from build123d import *

# Parameters (mm, degrees)
SKIZZE1_R                                            = 8
AUFSATZ_LINEAR_AUSTRAGEN1_DEPTH                      = 5
AUFSATZ_LINEAR_AUSTRAGEN2_DEPTH                      = 7.5
FORMSENKUNG_F_R_M3_SENKSCHRAUBE_MIT_SCHL_D           = 3.2
FORMSENKUNG_F_R_M3_SENKSCHRAUBE_MIT_SCHL_CSINK_D     = 6.3
FORMSENKUNG_F_R_M3_SENKSCHRAUBE_MIT_SCHL_CSINK_ANGLE = 90
M4_GEWINDEBOHRUNG2_D                                 = 3.3
M4_GEWINDEBOHRUNG2_DEPTH                             = 13
M4_GEWINDEBOHRUNG2_TIP                               = 0.991420021
SKIZZE15_R                                           = 18.25
SCHNITT_LINEAR_AUSTRAGEN1_DEPTH                      = 1
SKIZZE16_R                                           = 11.0125
SCHNITT_LINEAR_AUSTRAGEN2_DEPTH                      = 2.5


with BuildPart() as part:
    # Skizze1 → Aufsatz-Linear austragen1 (new body)
    with BuildSketch(Plane.XY):
        with BuildLine():
            Line((0, 0), (52.5, 0))
            Line((52.5, 0), (52.5, 7.5))
            Line((52.5, 7.5), (48.11327046, 38.207106781))
            ThreePointArc((48.11327046, 38.207106781), (46.439531698, 41.277269775), (43.163522992, 42.5))
            Line((43.163522992, 42.5), (9.336477008, 42.5))
            ThreePointArc((9.336477008, 42.5), (6.060468302, 41.277269775), (4.38672954, 38.207106781))
            Line((4.38672954, 38.207106781), (0, 7.5))
            Line((0, 7.5), (0, 0))
        make_face()
        with Locations((26.25, 21.25)):
            Circle(SKIZZE1_R, mode=Mode.SUBTRACT)
    extrude(amount=AUFSATZ_LINEAR_AUSTRAGEN1_DEPTH)

    # Skizze4 → Aufsatz-Linear austragen2 (add)
    with BuildSketch(Plane.XZ):
        with BuildLine():
            Line((52.5, 0), (47.5, 0))
            Line((47.5, 0), (47.5, -7.5))
            ThreePointArc((47.5, -7.5), (50, -10), (52.5, -7.5))
            Line((52.5, -7.5), (52.5, 0))
        make_face()
        with BuildLine():
            Line((0, 0), (5, 0))
            Line((5, 0), (5, -7.5))
            ThreePointArc((5, -7.5), (2.5, -10), (0, -7.5))
            Line((0, -7.5), (0, 0))
        make_face()
    extrude(amount=-AUFSATZ_LINEAR_AUSTRAGEN2_DEPTH)

    # Formsenkung für M3 Senkschraube mit Schlitz/Kreuzschlitz1 (through all)
    with Locations(Plane.XY.offset(5)):
        with Locations((16.350505063, 31.149494937), (36.149494937, 11.350505063), (16.350505063, 11.350505063), (36.149494937, 31.149494937)):
            CounterSinkHole(FORMSENKUNG_F_R_M3_SENKSCHRAUBE_MIT_SCHL_D / 2, FORMSENKUNG_F_R_M3_SENKSCHRAUBE_MIT_SCHL_CSINK_D / 2, counter_sink_angle=FORMSENKUNG_F_R_M3_SENKSCHRAUBE_MIT_SCHL_CSINK_ANGLE)

    # M4 Gewindebohrung2
    with Locations(Plane(origin=(0, 0, 0), x_dir=(-1, 0, 0), z_dir=(0, -1, 0))):
        with Locations((-2.5, 7.5), (-50, 7.5), (-50, -2.5), (-2.5, -2.5)):
            Hole(M4_GEWINDEBOHRUNG2_D / 2, depth=M4_GEWINDEBOHRUNG2_DEPTH)
            with Locations((0, 0, -(M4_GEWINDEBOHRUNG2_DEPTH + M4_GEWINDEBOHRUNG2_TIP / 2))):  # 118° drill point
                Cone(0, M4_GEWINDEBOHRUNG2_D / 2, M4_GEWINDEBOHRUNG2_TIP, mode=Mode.SUBTRACT)

    # Skizze15 → Schnitt-Linear austragen1 (cut)
    with BuildSketch(Plane(origin=(0, 0, 0), x_dir=(-1, 0, 0), z_dir=(0, 0, -1))):
        with Locations((-26.25, 21.25)):
            Circle(SKIZZE15_R)
    extrude(amount=-SCHNITT_LINEAR_AUSTRAGEN1_DEPTH, mode=Mode.SUBTRACT)

    # Skizze16 → Schnitt-Linear austragen2 (cut)
    with BuildSketch(Plane(origin=(0, 0, 1), x_dir=(-1, 0, 0), z_dir=(0, 0, -1))):
        with Locations((-26.25, 21.25)):
            Circle(SKIZZE16_R)
    extrude(amount=-SCHNITT_LINEAR_AUSTRAGEN2_DEPTH, mode=Mode.SUBTRACT)


solid = part.part
Source: CAD feature listing. Evaluate the final solid. Frame: model axes, mm. A direction names the side the tool comes from. Give positions to 0.01 mm unless a question says otherwise; leave off trailing zeros. Write each loop counter-clockwise with the first axis right and the second up, starting at its lowest first coordinate (ties: lowest second). Pieces come first, ordered by that corner, then holes. Notation, with made-up numbers: (72.5, 40.25) - (88.5, 40.25) arc R26 ccw to (88.5, 62.25) - close; hole circle Ø5 at (56.25, 52.25). An arc over 180 degrees is marked (long way). Write item = value, one per line. Start each with the question number.
Q1. Reachability of faces 4 (the flat face through (19, 25, 3.5)), 5 (the cylindrical face through (6.1, 41.31, 2.46)), 6 (the flat face through (3, 7.5, -4)), 7 (the flat face through (0, 4, -1)), 8 (the cylindrical face through (48.35, 6.59, 2.43)) from +Z, -Z, +X, -X, +Y, -Y: full face, straight path, thin tool, end or side. Return the list, or none.
Q2. Draft query along Y for faces 1 (the cylindrical face through (39.701, 33.584, 0.493)), 2 (the flat face through (2.224, 23.069, 2.465)), 3 (the flat face through (52.5, 4, -1)). Return one class per face: +Y half, -Y half, draft (parallel to the pull), parting line (faces both ways), or undercut.
Q3. Pin query (flat end, axial travel): pin 1 Ø4 at (x, y) = (36.15, 11.35) entering from -Z; pin 2 Ø3 at (x, y) = (16.35, 31.15) entering from +Z; pin 3 Ø17.5 at (x, y) = (26.25, 21.25) entering from -Z; pin 4 Ø5.5 at (x, z) = (50, -7.5) entering from -Y. Return the tip coordinate at first contact, or that it passes through.
Q4. Material intervals for probe 1 along X at (y, z) = (5, -7.5); probe 2 along X at (y, z) = (4, -4.5); probe 3 along X at (y, z) = (3, 1), sorted ascending.
Q5. Cut plane A-A, the plane z = -2.5. Return loops of the section in (x, y).
Q6. Cut plane C-C, the plane y = 21.25. Return loops of the section in (x, z), then the cut area to 3 significant figures.
Q7. Cut plane B-B, the plane x = 22.5. Return loops of the section in (y, z).
Computed values:
q1.face_4 = -Z
q1.face_5 = +Z, -Z, -X, +Y
q1.face_6 = -Z, +X, -X, +Y
q1.face_7 = +Z, -Z, -X, +Y, -Y
q1.face_8 = -Y
q2.face_1 = undercut
q2.face_2 = +Y half
q2.face_3 = draft
q3.pin_1 = 1
q3.pin_2 = through
q3.pin_3 = 3.5
q3.pin_4 = 0
q4.probe_1 = 0 to 0.85, 4.15 to 5, 47.5 to 48.35, 51.65 to 52.5
q4.probe_2 = 0 to 5, 47.5 to 52.5
q4.probe_3 = 0 to 1.81, 3.19 to 49.31, 50.69 to 52.5
q5.outline = (0, 0) - (5, 0) - (5, 7.5) - (0, 7.5) - close; (47.5, 0) - (52.5, 0) - (52.5, 7.5) - (47.5, 7.5) - close
q6.outline = (1.96, 0) - (8, 0) - (8, 1) - (15.24, 1) - (15.24, 3.5) - (18.25, 3.5) - (18.25, 5) - (1.96, 5) - close; (34.25, 3.5) - (37.26, 3.5) - (37.26, 1) - (44.5, 1) - (44.5, 0) - (50.54, 0) - (50.54, 5) - (34.25, 5) - close
q6.area = 127 mm²
q7.outline = (0, 0) - (3.39, 0) - (3.39, 1) - (10.9, 1) - (10.9, 3.5) - (14.18, 3.5) - (14.18, 5) - (0, 5) - close; (28.32, 3.5) - (31.6, 3.5) - (31.6, 1) - (39.11, 1) - (39.11, 0) - (42.5, 0) - (42.5, 5) - (28.32, 5) - close
